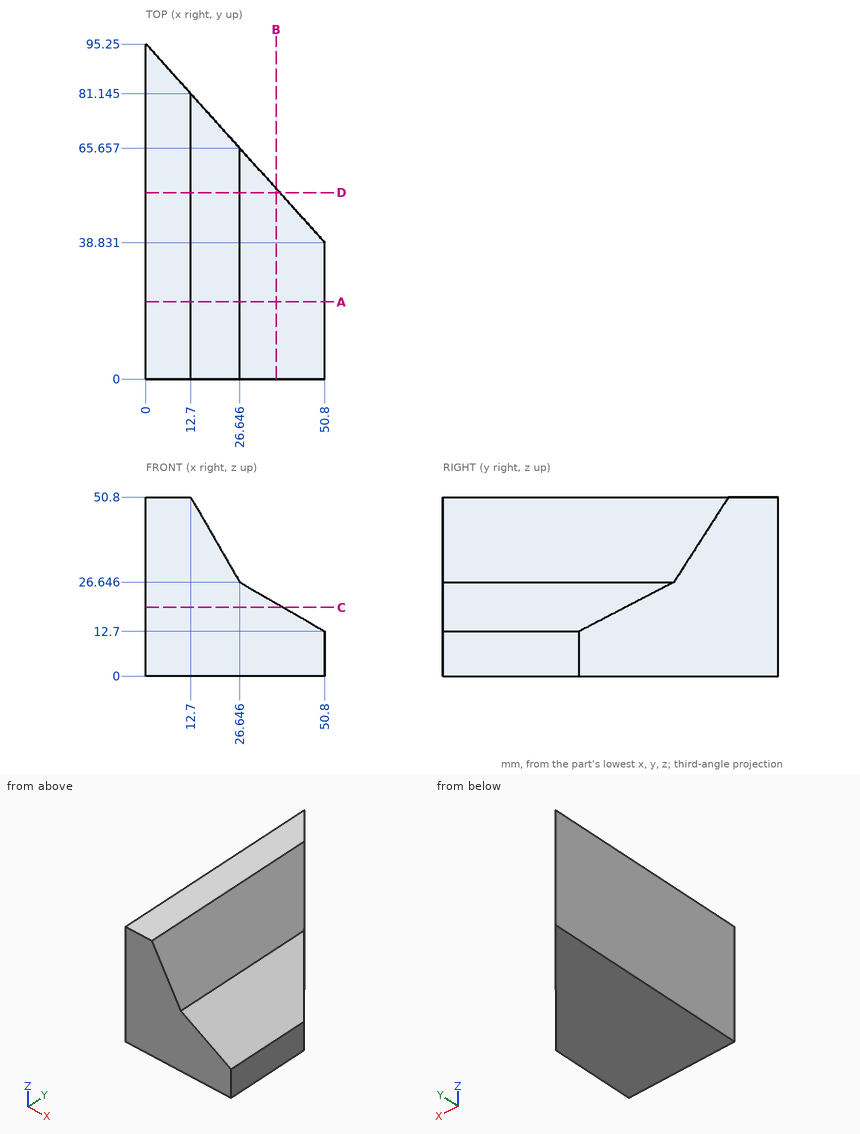
Print and shaded views of the part. All mm, measured from the part's lowest x, y and z. Give positions to 0.01 mm unless a question says otherwise; leave off trailing zeros. Write each loop counter-clockwise with the first axis right and the second up, starting at its lowest first coordinate (ties: lowest second). Pieces come first, ordered by that corner, then holes. Notation, with made-up numbers: (84, -26) -> (121, -26) arc R19 ccw to (121, -10) -> close; hole circle Ø10 at (56, -6). An arc over 180 degrees is marked (long way). Use CSV: the item, a comma, the result in double quotes. Start each with the question number.
1) Pin check, flat tips, straight feed: P1, Ø4, axis at y = 50, z = 20, coming from the +X side; P2, Ø8, axis at y = 58, z = 23, coming from the +X side; P3, Ø12, axis at x = 15.5, z = 25, coming from the +Y side. Stop position of each tip, or through.
2) Cut at D-D on y = 53. List the corners of the cut face in (x, z) (1 decimal), plus the area to 3 significant figures.
3) Cut at B-B on x = 37. List the corners of the cut face in (y, z).
4) Drill centre lines: L1, parallel to Y at x = 9.5, z = 25.5; L2, parallel to Z at x = 33.5, y = 8; L3, parallel to Y at x = 10, z = 44 (1 decimal). Where is each one in solid material? Low to high.
5) Cut at A-A on y = 22. List the corners of the cut face in (x, z) (1 decimal).
6) Cut at C-C on z = 19.5. List the corners of the cut face in (x, y).
Final values:
1,P1,"stops at x = 41.39"
1,P2,"stops at x = 36.6"
1,P3,"stops at y = 84.7"
2,outline,"(0, 0) -> (38, 0) -> (38, 20.1) -> (26.6, 26.6) -> (12.7, 50.8) -> (0, 50.8) -> close"
2,area,"1,450 mm2"
3,outline,"(0, 0) -> (54.16, 0) -> (54.16, 20.67) -> (0, 20.67) -> close"
4,L1,"y = 0 to 84.7"
4,L2,"z = 0 to 22.69"
4,L3,"y = 0 to 84.1"
5,outline,"(0, 0) -> (50.8, 0) -> (50.8, 12.7) -> (26.6, 26.6) -> (12.7, 50.8) -> (0, 50.8) -> close"
6,outline,"(0, 0) -> (39.02, 0) -> (39.02, 51.91) -> (0, 95.25) -> close"
